```python
from build123d import *

# Parameters (mm, degrees)
F0_R     = 12
F1_DEPTH = 40
F3_DEPTH = 15


with BuildPart() as f1:
    # F0 (on Top) → F1 (new body)
    with BuildSketch(Plane.XY):
        Circle(F0_R)
    extrude(amount=F1_DEPTH)

    # F2 (on Top) → F3 (join)
    with BuildSketch(Plane.XY):
        Polygon((20.78461, 0), (10.392305, 18), (-10.392305, 18), (-20.78461, 0), (-10.392305, -18), (10.392305, -18), align=None)
    extrude(amount=-F3_DEPTH)


solid = f1.part
```
Work out the finished part from the listing and answer in its coordinate system (mm). A direction names the side the tool comes from. Give positions to 0.01 mm unless a question says otherwise; leave off trailing zeros. Loops run counter-clockwise (first coordinate to the right, second up) from the corner with the lowest first, then second, coordinate; pieces in that order, holes last. Notation, with made-up numbers: (-4.5, -3.5) -> (43.5, -3.5) arc R21 cw to (43.5, 4.5) -> close; hole circle Ø5 at (9, 88). An arc over 180 degrees is marked (long way). Put each result on its own line as item: value. Start each with the question number.
Item 1: The part is cut by section B-B (y = 3). Give the vertices of the cut face in (x, z).
Item 2: Find the intervals of material crossed by L1, parallel to Y at x = -6, z = 21; L2, parallel to Z at x = -13, y = 4.5; L3, parallel to X at y = -2, z = -0.5, in increasing order. Write a range as [from, to].
Item 3: The part is cut by section C-C (z = -9). Give the vertices of the cut face in (x, y).
Item 4: The part is cut by section D-D (z = 10). Give the vertices of the cut face in (x, y), then the cut area to 3 significant figures.
Item 5: The part is cut by section A-A (x = 0). Give the vertices of the cut face in (y, z).
Item 6: Each of these flat-tipped pins is pushed along its axis until it touches: P1, Ø4, axis at y = 2.5, z = 16, coming from the -X side; P2, Ø3, axis at x = 12.5, z = 12, coming from the +Y side; P3, Ø1, axis at x = 7, z = 4.5, coming from the -Y side. Where does it stop, or does it pass through?
Item 7: Which of the six approach directions +Z, -Z, +X, -X, +Y, -Y give full straight-line access (tool end or side, diameter ignored) to faces 1 (the face through (-11.99, 0.53, 19.72)), 2 (the face through (0, 0, 40))?
Answers below:
1. outline: (-19.05, -15) -> (19.05, -15) -> (19.05, 0) -> (11.62, 0) -> (11.62, 40) -> (-11.62, 40) -> (-11.62, 0) -> (-19.05, 0) -> close
2. L1: [-10.39, 10.39]
2. L2: [-15, 0]
2. L3: [-19.63, 19.63]
3. outline: (-20.78, 0) -> (-10.39, -18) -> (10.39, -18) -> (20.78, 0) -> (10.39, 18) -> (-10.39, 18) -> close
4. outline: circle Ø24 at (0, 0)
4. area: 452 mm2
5. outline: (-18, -15) -> (18, -15) -> (18, 0) -> (12, 0) -> (12, 40) -> (-12, 40) -> (-12, 0) -> (-18, 0) -> close
6. P1: x = -11.99
6. P2: y = 4.8
6. P3: y = -10.09
7. face 1: +Z
7. face 2: +Z, +X, -X, +Y, -Y
